Study the drawing (mm; zero at the part's minimum x, y, z) and answer. Round coordinates to 2 decimals unless told otherwise and drop trailing zeros. Loops run counter-clockwise (first coordinate to the right, second up) from the corner with the lowest first, then second, coordinate; pieces in that order, holes last. Notation, with made-up numbers: M 71.25,-9.75 L 82.25,-9.75 A25 cw 82.25,26.25 Z; hole C -16.75,3 d10. An arc over 180 degrees is marked long. Write each question's results on one line, items separated by ' | '.
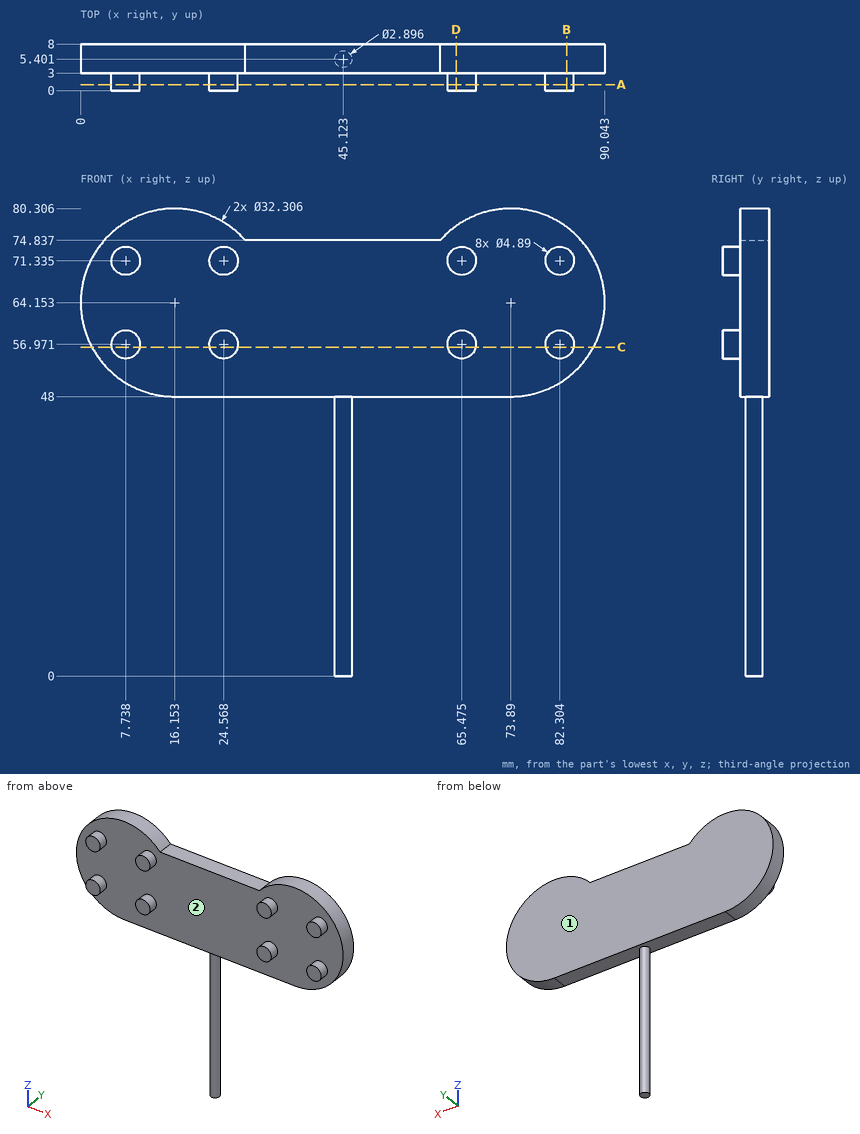
Item 1: Straight lines are drawn through the part: line 1 (Z direction, x = 39.5, y = 3.5); line 2 (Y direction, x = 14.5, z = 74); line 3 (X direction, y = 5, z = 65). For each, find the intervals that lie inside material, in ascending order.
Outcome:
line 1: z = 48 to 74.84 | line 2: y = 3 to 8 | line 3: x = 0.02 to 90.02
Item 2: The part is cut by section B-B (x = 83.5). Determine the outline of the cut face in (y, z), plus the area to 3 significant figures.
Outcome:
outline: M 0,54.84 L 3,54.84 L 3,51.17 L 8,51.17 L 8,77.14 L 3,77.14 L 3,73.47 L 0,73.47 L 0,69.2 L 3,69.2 L 3,59.1 L 0,59.1 Z | area: 155 mm2
Item 3: The part is cut by section D-D (x = 64.5). Determine the outline of the cut face in (y, z).
Outcome:
outline: M 0,54.73 L 3,54.73 L 3,48 L 8,48 L 8,77.3 L 3,77.3 L 3,73.58 L 0,73.58 L 0,69.09 L 3,69.09 L 3,59.21 L 0,59.21 Z
Item 4: The part is cut by section A-A (y = 1). Determine the outline of the cut face in (x, z) (1 decimal).
Outcome:
outline: C 7.7,57 d4.9; C 7.7,71.3 d4.9; C 24.6,57 d4.9; C 24.6,71.3 d4.9; C 65.5,57 d4.9; C 65.5,71.3 d4.9; C 82.3,57 d4.9; C 82.3,71.3 d4.9
Item 5: Flat-ended cylindrical pins translate along their axes: pin 1 (4 mm diameter, centred on x = 53.5, y = 5.5, fed in from +Z); pin 2 (3 mm diameter, centred on x = 31, y = 2, fed in from -Z); pin 3 (4 mm diameter, centred on y = 2, z = 49, fed in from +X). Find the tip coordinate at first contact, or state that the pin passes through.
Outcome:
pin 1: stops at z = 74.84 | pin 2: stops at z = 48 | pin 3: stops at x = 82.88
Item 6: The part is cut by section C-C (z = 56.5). Determine the outline of the cut face in (x, y) (1 decimal).
Outcome:
outline: M 1.9,3 L 5.3,3 L 5.3,0 L 10.1,0 L 10.1,3 L 22.2,3 L 22.2,0 L 27,0 L 27,3 L 63.1,3 L 63.1,0 L 67.9,0 L 67.9,3 L 79.9,3 L 79.9,0 L 84.7,0 L 84.7,3 L 88.1,3 L 88.1,8 L 1.9,8 Z
Item 7: The mould has two halves that part along X. Classify the marked faces 1 and 2: pulls with the +X half, pulls with the -X half, needs draft (parallel to the pull), parting line crosses it, or undercut.
Outcome:
face 1: needs draft | face 2: undercut
